Design review of the part shown in the three views and the two pictorial views. Dimensions are in mm from the part's minimum x, y and z. A direction names the side the tool comes from. Give positions to 0.01 mm unless a question says otherwise; leave off trailing zeros. Order: outer loops, then holes, each group sorted by start corner. A loop starts at its lowest first (then second) coordinate and runs counter-clockwise, first axis right, second up.
Item 1: Consider section A-A (z = 63.5). Give the boundary of the cut face in (x, y).
Item 2: Consider section C-C (y = 25). Give the boundary of the cut face in (x, z), plus the area to 3 significant figures.
Item 3: For P1, Ø7, axis at x = 13.5, y = 55.5, coming from the -Z side; P2, Ø1.9, axis at x = 4, z = 55, coming from the +Y side; P3, Ø6.5, axis at x = 14.5, z = 57, coming from the +Y side; P4, Ø12, axis at x = 10, y = 27, coming from the -Z side, all flat-tipped, find the tip position at first contact; note any pin that passes through.
Item 4: Machinability: for the marked faces 1, 2, 3 and 4, which of the approach directions +Z, -Z, +X, -X, +Y, -Y give a long, thin tool a straight path to every point of the face, cutting with its end or side? Answer none if there is none.
Item 5: For probe 1 along Y at (x, z) = (13.75, 38.1) (3 decimals); probe 2 along Z at (x, y) = (14.5, 69.85) (3 decimals); probe 3 along Y at (x, z) = (2, 61.5), list the stretches that pass through material, from the lowest coordinate up.
Item 6: Consider section B-B (x = 20.75). Give the boundary of the cut face in (y, z), plus the area to 3 significant figures.
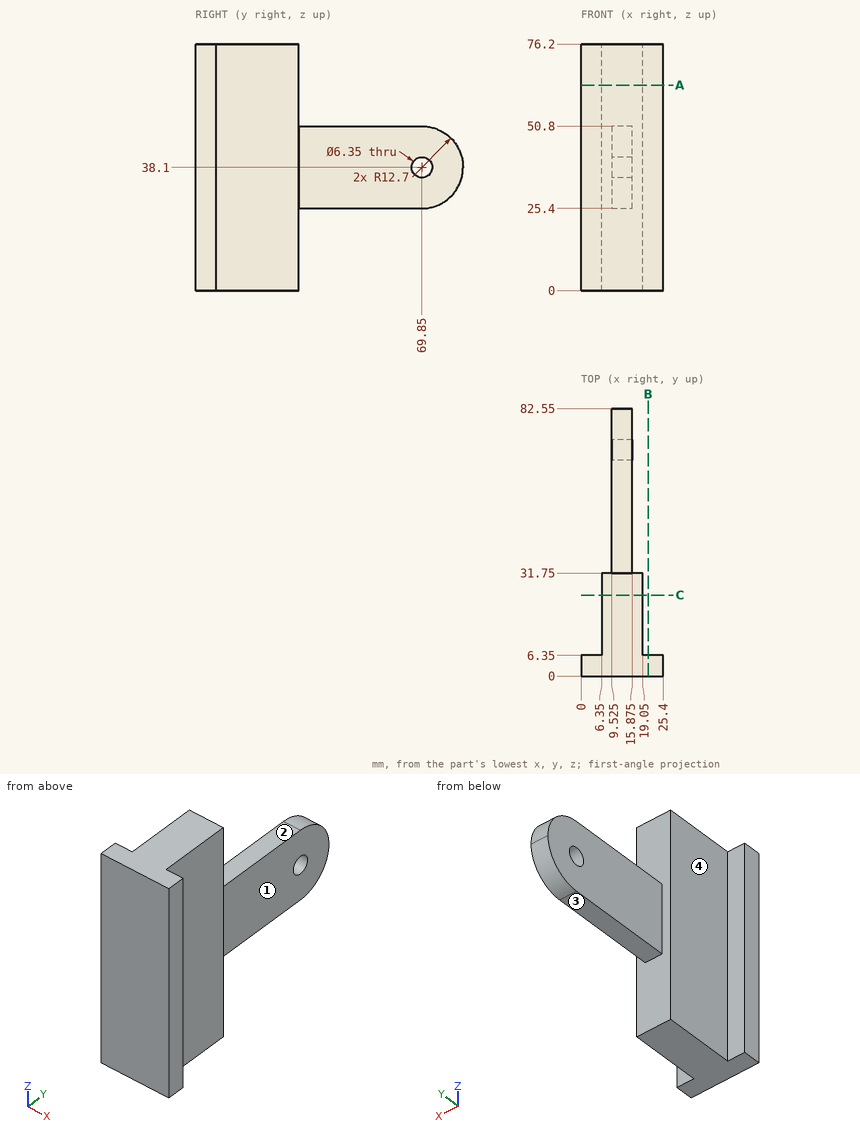
Resolved:
1. outline: (0, 0) - (25.4, 0) - (25.4, 6.35) - (19.05, 6.35) - (19.05, 31.75) - (6.35, 31.75) - (6.35, 6.35) - (0, 6.35) - close
2. outline: (6.35, 0) - (19.05, 0) - (19.05, 76.2) - (6.35, 76.2) - close
2. area: 968 mm2
3. P1: stops at z = 25.4
3. P2: stops at y = 6.35
3. P3: stops at y = 31.75
3. P4: stops at z = 0
4. face 1: +Z, -Z, +X, +Y
4. face 2: +Z, +X, -X, +Y
4. face 3: -Z, +X, -X, +Y
4. face 4: +Z, -Z, -X, +Y
5. probe 1: y = 0 to 66.675, 73.025 to 82.55
5. probe 2: z = 25.4 to 34.925, 41.275 to 50.8
5. probe 3: y = 0 to 6.35
6. outline: (0, 0) - (6.35, 0) - (6.35, 76.2) - (0, 76.2) - close
6. area: 484 mm2
